Autodesk Fusion 360 part; units mm, degrees
sketch "Sketch1" plane through (0, 0, 0) normal (0, 0, 1) x (1, 0, 0)
  line L0 (6.375, 3.625) -> (-6.375, 3.625)
  line L1 (-6.375, 3.625) -> (-6.375, -3.625)
  line L2 (-6.375, -3.625) -> (6.375, -3.625)
  line L3 (6.375, -3.625) -> (6.375, 3.625)
  line L4 (6.375, 3.625) -> (-6.375, -3.625) construction
  line L5 (-6.375, 3.625) -> (6.375, -3.625) construction
  line L6 (33.25, -12.5) -> (-33.25, -12.5)
  line L7 (-33.25, -12.5) -> (-33.25, 12.5)
  line L8 (-33.25, 12.5) -> (33.25, 12.5)
  line L9 (33.25, 12.5) -> (33.25, -12.5)
  line L10 (33.25, -12.5) -> (-33.25, 12.5) construction
  line L11 (-33.25, -12.5) -> (33.25, 12.5) construction
  line L12 (-33.25, -12.5) -> (-40.25, -12.5)
  line L13 (-40.25, -12.5) -> (-40.25, 12.5)
  line L14 (-40.25, 12.5) -> (-33.25, 12.5)
  line L15 (-33.25, 12.5) -> (-33.25, -12.5)
  line L16 (0, 1.75) -> (0, 22.5)
  line L17 (40.25, -12.5) -> (40.25, 12.5)
  line L18 (40.25, 12.5) -> (33.25, 12.5)
  line L19 (33.25, -12.5) -> (33.25, 12.5)
  line L20 (33.25, -12.5) -> (40.25, -12.5)
  dimension "d1" = 12.75
  dimension "d2" = 7.25
  dimension "d3" = 25
  dimension "d4" = 66.5
  dimension "d7" = 7
  dimension "d8" = 25
extrude "Extrude1" add sketch "Sketch1" along normal blind 8 contours L6 L7 L8 L9 L15 L19
extrude "Extrude2" add sketch "Sketch1" along normal blind 48 contours L7 L12 L13 L14 L15 | L9 L17 L18 L19 L20
sketch "Sketch2" plane through (0, 0, 48) normal (0, 0, 1) x (-1, 0, 0)
  line L0 (33.25, -12.5) -> (40.25, -12.5)
  line L1 (40.25, -12.5) -> (40.25, 12.5)
  line L2 (40.25, 12.5) -> (33.25, 12.5)
  line L3 (33.25, 12.5) -> (33.25, -12.5)
  line L4 (40.25, 12.5) -> (60.25, 12.5)
  line L5 (60.25, 12.5) -> (60.25, -12.5)
  line L6 (60.25, -12.5) -> (40.25, -12.5)
  line L7 (40.25, -12.5) -> (40.25, 12.5)
  circle A0 centre (50.25, 0) radius 1.7
  line L8 (60.25, 0) -> (40.25, 0)
  line L9 (0, -1.75) -> (0, -22.5)
  line L10 (-60.25, 12.5) -> (-60.25, -12.5)
  line L11 (-60.25, -12.5) -> (-40.25, -12.5)
  line L12 (-40.25, -12.5) -> (-40.25, 12.5)
  line L13 (-40.25, 12.5) -> (-60.25, 12.5)
  line L14 (-60.25, 0) -> (-40.25, 0)
  circle A1 centre (-50.25, 0) radius 1.7
  dimension "d11" = 20
  dimension "d12" = 3.4
  dimension "d13" = 25
extrude "Extrude3" add sketch "Sketch2" against normal blind 5 contours L1 L5 L6 L7 A0 L8 | L1 L4 L5 L7 A0 L8 | L10 L12 L13 L14 A1 | L10 L11 L12 L14 A1
chamfer "Chamfer1" distance 2 angle 45 2 edges at (-48.665, 0.6147, 43) (51.835, 0.6147, 43)
fillet "Fillet3" radius 5 4 edges at (40.25, 0, 0) (-40.25, 0, 0) (-40.25, 0, 43) (40.25, 0, 43)
fillet "Fillet4" radius 1 4 edges at (-33.25, 0, 8) (33.25, 0, 8) (33.25, 0, 48) (-33.25, 0, 48)
chamfer "Chamfer2" distance 5 angle 45 4 edges at (-60.25, 12.5, 45.5) (-60.25, -12.5, 45.5) (60.25, -12.5, 45.5) (60.25, 12.5, 45.5)
sketch "Sketch3" plane through (0, -12.5, 0) normal (0, -1, 0) x (1, 0, 0)
  line L0 (55.25, 43) -> (55.25, 48)
  line L1 (55.25, 48) -> (34.25, 48)
  arc A0 (34.25, 48) -> (33.25, 47) centre (34.25, 47) ccw
  line L2 (33.25, 47) -> (33.25, 9)
  arc A1 (32.25, 8) -> (33.25, 9) centre (32.25, 9) ccw
  line L3 (32.25, 8) -> (-32.25, 8)
  arc A2 (-33.25, 9) -> (-32.25, 8) centre (-32.25, 9) ccw
  line L4 (-33.25, 9) -> (-33.25, 47)
  arc A3 (-33.25, 47) -> (-34.25, 48) centre (-34.25, 47) ccw
  line L5 (-34.25, 48) -> (-55.25, 48)
  line L6 (-55.25, 48) -> (-55.25, 43)
  line L7 (-55.25, 43) -> (-45.25, 43)
  arc A4 (-40.25, 38) -> (-45.25, 43) centre (-45.25, 38) ccw
  line L8 (-40.25, 38) -> (-40.25, 5)
  arc A5 (-40.25, 5) -> (-35.25, 0) centre (-35.25, 5) ccw
  line L9 (-35.25, 0) -> (35.25, 0)
  arc A6 (35.25, 0) -> (40.25, 5) centre (35.25, 5) ccw
  line L10 (40.25, 5) -> (40.25, 38)
  arc A7 (45.25, 43) -> (40.25, 38) centre (45.25, 38) ccw
  line L11 (45.25, 43) -> (55.25, 43)
  line L12 (-6.375, 0) -> (6.375, 0)
  line L13 (6.375, 0) -> (6.375, 8)
  line L14 (6.375, 8) -> (-6.375, 8)
  line L15 (-6.375, 8) -> (-6.375, 0)
  line L16 (0, 4) -> (0, 0) construction
  line L17 (0, 4) -> (-6.375, 4) construction
  circle A8 centre (0, 4) radius 1.3
  dimension "d39" = 2.6
extrude "Extrude4" cut sketch "Sketch3" against normal blind 8.875 contours A8
equation "d3 = thickness"
equation "d8 = d3"
equation "d13 = thickness"
equation "thickness = 25 mm"
Verification items for the finished model (mm, model axes). A direction names the side the tool comes from. Coordinates: 2 decimals unless noted, no trailing zeros. Loops run counter-clockwise (first coordinate to the right, second up) from the corner with the lowest first, then second, coordinate; pieces in that order, holes last. Notation, with made-up numbers: (-10.75, 82) - (45.25, 82) arc R31 cw to (45.25, 107) - close; hole circle Ø3 at (-8, -18). An arc over 180 degrees is marked (long way). Put each result on its own line as item: value.
Item 1: Section check A-A (x = 3). Enter the section's corners in (y, z) (3 decimals).
Conclusion:
outline: (-12.5, 0) - (-3.625, 0) - (-3.625, 8) - (-12.5, 8) - close; (3.625, 0) - (12.5, 0) - (12.5, 8) - (3.625, 8) - close
Item 2: Set-up check for faces 4 (the face through (-51.94, -0.7, 44.87)), 5 (the face through (-57.785, 9.965, 45.465)), 6 (the face through (-33.25, 0, 28)), 7 (the face through (55, 0, 43)), 8 (the face through (-40.25, 0, 21)): record each of +Z, -Z, +X, -X, +Y, -Y from which the full face is reachable in a straight line by a thin tool's end or side.
Conclusion:
face 4: -Z
face 5: +Z, -Z, -X, +Y
face 6: +Z, +Y, -Y
face 7: -Z, +X, +Y, -Y
face 8: -Z, -X, +Y, -Y
Item 3: Section check B-B (z = 28.5). Enter the section's corners in (x, y), then the cut area to 3 significant figures.
Conclusion:
outline: (-40.25, -12.5) - (-33.25, -12.5) - (-33.25, 12.5) - (-40.25, 12.5) - close; (33.25, -12.5) - (40.25, -12.5) - (40.25, 12.5) - (33.25, 12.5) - close
area: 350 mm2
Item 4: Scan lines: line 1 along X through (y, z) = (0, 46); line 2 along X through (y, z) = (0, 47.2); line 3 along X through (y, z) = (-1, 15.5). Record each from-to range of solid material in increasing order.
Conclusion:
line 1: x = -60.25 to -51.95, -48.55 to -33.25, 33.25 to 48.55, 51.95 to 60.25
line 2: x = -60.25 to -51.95, -48.55 to -33.27, 33.27 to 48.55, 51.95 to 60.25
line 3: x = -40.25 to -33.25, 33.25 to 40.25
Item 5: Draft check along Y on faces 1 (the face through (0.8, -12.5, 7.7)), 2 (the face through (-38.75, 0.18, 1.43)), 3 (the face through (-6.375, 0, 4)). Enter one of: pulls with the +Y half, pulls with the -Y half, needs draft (parallel to the pull), parting line crosses it, or undercut.
Conclusion:
face 1: pulls with the -Y half
face 2: needs draft
face 3: undercut
Item 6: Section check C-C (y = -9). Enter the section's corners in (x, z), then the cut area to 3 significant figures.
Conclusion:
outline: (-58.75, 43) - (-45.25, 43) arc R5 cw to (-40.25, 38) - (-40.25, 5) arc R5 ccw to (-35.25, 0) - (35.25, 0) arc R5 ccw to (40.25, 5) - (40.25, 38) arc R5 cw to (45.25, 43) - (58.75, 43) - (58.75, 48) - (34.25, 48) arc R1 ccw to (33.25, 47) - (33.25, 9) arc R1 cw to (32.25, 8) - (-32.25, 8) arc R1 cw to (-33.25, 9) - (-33.25, 47) arc R1 ccw to (-34.25, 48) - (-58.75, 48) - close; hole circle Ø2.6 at (0, 4)
area: 1,380 mm2
Item 7: Section check D-D (y = 0). Give the number of separate pieces and of enclosed holes in the cut face, then the cut area to 3 significant figures.
Conclusion:
separate pieces: 4
enclosed holes: 0
area: 1,260 mm2
Item 8: Gauge pin test, flat ends, axial feed: pin 1 Ø7.5 at (x, y) = (-56, 0.5) entering from -Z; pin 2 Ø3.5 at (y, z) = (0.5, 5.5) entering from +X; pin 3 Ø4 at (x, y) = (37.5, 1) entering from -Z. Record the tip position at first contact, or that the pin passes through.
Conclusion:
pin 1: stops at z = 43
pin 2: stops at x = 40.25
pin 3: stops at z = 0.01
